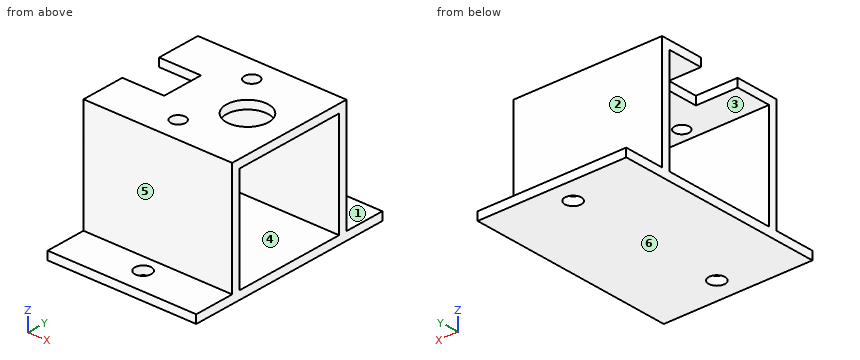
```python
from build123d import *

# Parameters (mm, degrees)
SKETCH072_W     = 35.5
SKETCH072_H     = 31.05
PAD050_DEPTH    = 2
SKETCH073_W     = 35.5
SKETCH073_H     = 2
PAD051_DEPTH    = 25
SKETCH074_R     = 1.95
PAD052_DEPTH    = 2
SKETCH075_R     = 1.75
SKETCH075_R_2   = 5
SKETCH075_W     = 10
SKETCH075_H     = 10
POCKET013_DEPTH = 2


with BuildPart() as part:
    # Sketch072 → Pad050 (new body)
    with BuildSketch(Plane.XY):
        Rectangle(SKETCH072_W, SKETCH072_H)
    extrude(amount=PAD050_DEPTH)

    # Sketch073 (on Face5 of Pad050) → Pad051 (join)
    with BuildSketch(Plane(origin=(0, 0, 0), x_dir=(1, 0, 0), z_dir=(0, 0, -1))):
        with Locations((0, 14.525)):
            Rectangle(SKETCH073_W, SKETCH073_H)
        with Locations((0, -14.525)):
            Rectangle(SKETCH073_W, SKETCH073_H)
    extrude(amount=PAD051_DEPTH)

    # Sketch074 (on Face16 of Pad051) → Pad052 (join)
    with BuildSketch(Plane(origin=(0, 0, -25), x_dir=(1, 0, 0), z_dir=(0, 0, -1))):
        Polygon((-17.75, 25.275), (17.75, 25.275), (17.75, 15.525), (17.75, -15.525), (17.75, -25.275), (-17.75, -25.275), (-17.75, -15.525), (-17.75, 15.525), align=None)
        with Locations((0, 19.525)):
            Circle(SKETCH074_R, mode=Mode.SUBTRACT)
        with Locations((0, -19.525)):
            Circle(SKETCH074_R, mode=Mode.SUBTRACT)
    extrude(amount=PAD052_DEPTH)

    # Sketch075 (on Face6 of Pad050) → Pocket013 (cut)
    with BuildSketch(Plane.XY.offset(2)):
        with Locations((0, 10)):
            Circle(SKETCH075_R)
        with Locations((0, -10)):
            Circle(SKETCH075_R)
        with Locations((7.75, 0)):
            Circle(SKETCH075_R_2)
        with Locations((-12.75, 0)):
            Rectangle(SKETCH075_W, SKETCH075_H)
    extrude(amount=-POCKET013_DEPTH, mode=Mode.SUBTRACT)


with BuildPart() as part_1:
    # Body017 placement: moved
    add(part.part.moved(Location((40, 0, -2))))


solid = part_1.part
```
Design review of the part built by this model. Coordinates are the model's own, in mm. Face numbers are marked on the shaded views. A direction names the side the tool comes from. Give positions to 0.01 mm unless a question says otherwise; leave off trailing zeros. Write each loop counter-clockwise with the first axis right and the second up, starting at its lowest first coordinate (ties: lowest second). Pieces come first, ordered by that corner, then holes. Notation, with made-up numbers: (-26, 65) -> (7, 65) arc R19 ccw to (7, 84) -> close; hole circle Ø10 at (-32, 89.25). An arc over 180 degrees is marked (long way). Answer in a Markdown table with one row per item.
(1) To check wall thickness, follow probe 1 along Y at (x, z) = (40, -28.2) (3 decimals); probe 2 along Y at (x, z) = (40, -1.4) (3 decimals); probe 3 along Y at (x, z) = (48.5, -5) (3 decimals). State the ranges of each line that lie inside material, in increasing order.
Results:
| item | result |
|---|---|
| probe 1 | -25.275 to -21.475, -17.575 to 17.575, 21.475 to 25.275 |
| probe 2 | -15.525 to -11.75, -8.25 to 8.25, 11.75 to 15.525 |
| probe 3 | -15.525 to -13.525, 13.525 to 15.525 |
(2) Consider section C-C (x = 40). State the section outline as (y, z) points (3 decimals).
Results:
| item | result |
|---|---|
| outline | (-25.275, -29) -> (-21.475, -29) -> (-21.475, -27) -> (-25.275, -27) -> close; (-17.575, -29) -> (17.575, -29) -> (17.575, -27) -> (15.525, -27) -> (15.525, 0) -> (11.75, 0) -> (11.75, -2) -> (13.525, -2) -> (13.525, -27) -> (-13.525, -27) -> (-13.525, -2) -> (-11.75, -2) -> (-11.75, 0) -> (-15.525, 0) -> (-15.525, -27) -> (-17.575, -27) -> close; (-8.25, -2) -> (8.25, -2) -> (8.25, 0) -> (-8.25, 0) -> close; (21.475, -29) -> (25.275, -29) -> (25.275, -27) -> (21.475, -27) -> close |
(3) Clearance check with flat-ended pins moving along their axes: pin 1 (12 mm diameter, centred on x = 33.5, z = -18, fed in from -Y) (3 decimals); pin 2 (3 mm diameter, centred on x = 40, y = -19.525, fed in from -Z); pin 3 (1 mm diameter, centred on y = -0.5, z = -1.5, fed in from -X); pin 4 (1.6 mm diameter, centred on x = 25, z = -1, fed in from +Y) (3 decimals). State where each tip first meets the part, or that it passes through.
Results:
| item | result |
|---|---|
| pin 1 | y = -15.525 |
| pin 2 | through |
| pin 3 | x = 32.25 |
| pin 4 | y = 15.525 |
(4) For the marked faces 4, 5 and 6, list the 3-axis set-ups (+Z, -Z, +X, -X, +Y, -Y) from which the entire face can be reached by the end or side of a thin tool; tool diameter is ignored.
Results:
| item | result |
|---|---|
| face 4 | +X, -X |
| face 5 | +Z, +X, -X, -Y |
| face 6 | -Z, +X, -X, +Y, -Y |
(5) Consider section A-A (z = -9.75). State the section outline as (x, y) points (3 decimals), then the cut area to 3 significant figures.
Results:
| item | result |
|---|---|
| outline | (22.25, -15.525) -> (57.75, -15.525) -> (57.75, -13.525) -> (22.25, -13.525) -> close; (22.25, 13.525) -> (57.75, 13.525) -> (57.75, 15.525) -> (22.25, 15.525) -> close |
| area | 142 mm2 |
(6) Consider section B-B (y = 10). State the section outline as (x, z) points.
Results:
| item | result |
|---|---|
| outline | (22.25, -29) -> (57.75, -29) -> (57.75, -27) -> (22.25, -27) -> close; (22.25, -2) -> (38.25, -2) -> (38.25, 0) -> (22.25, 0) -> close; (41.75, -2) -> (57.75, -2) -> (57.75, 0) -> (41.75, 0) -> close |
(7) Mouldability with a two-part tool opening along Z and no side actions: class the marked faces 1, 2 and 3 as +Z half, -Z half, draft (parallel to the pull), parting line (faces both ways), or undercut.
Results:
| item | result |
|---|---|
| face 1 | +Z half |
| face 2 | draft |
| face 3 | undercut |
(8) Consider section D-D (x = 47.75). State the section outline as (y, z) points (3 decimals).
Results:
| item | result |
|---|---|
| outline | (-25.275, -29) -> (25.275, -29) -> (25.275, -27) -> (15.525, -27) -> (15.525, 0) -> (5, 0) -> (5, -2) -> (13.525, -2) -> (13.525, -27) -> (-13.525, -27) -> (-13.525, -2) -> (-5, -2) -> (-5, 0) -> (-15.525, 0) -> (-15.525, -27) -> (-25.275, -27) -> close |
